```python
from build123d import *

# Parameters (mm, degrees)
SKETCH2_R          = 1.75
SKETCH2_R_2        = 4
SKETCH2_R_3        = 1
CUT_EXTRUDE5_DEPTH = 31.724582991
SKETCH2_7_R        = 10
CUT_EXTRUDE6_DEPTH = 7.5


with BuildPart() as part:
    # Sketch1 → Revolve2 (revolve)
    with BuildSketch(Plane.XY):
        Polygon((0, 12), (0, 0), (-20, 0), (-20, 5), (-17.5, 5), (-17.5, 12), align=None)
    revolve(axis=Axis((0, 12, 0), (0, -1, 0)))

    # Sketch2 → Cut-Extrude5 (cut, through all)
    with BuildSketch(Plane.XZ):
        with Locations((-7.340557342, -12.660927377)):
            Circle(SKETCH2_R)
        with Locations((14.5, 0)):
            Circle(SKETCH2_R)
        with Locations((-7.384963415, 12.584013803)):
            Circle(SKETCH2_R)
        Circle(SKETCH2_R_2)
        with Locations((0, 7)):
            Circle(SKETCH2_R_3)
        with Locations((-7, 0)):
            Circle(SKETCH2_R_3)
        with Locations((7, 0)):
            Circle(SKETCH2_R_3)
        with Locations((0, -7)):
            Circle(SKETCH2_R_3)
    extrude(amount=-CUT_EXTRUDE5_DEPTH, mode=Mode.SUBTRACT)

    # Sketch2_7 → Cut-Extrude6 (cut)
    with BuildSketch(Plane.XZ):
        Circle(SKETCH2_7_R)
    extrude(amount=-CUT_EXTRUDE6_DEPTH, mode=Mode.SUBTRACT)


solid = part.part
```
Here's how the part is built. I have some questions about the finished solid (model axes, mm). A direction names the side the tool comes from. Coordinates: 2 decimals unless noted, no trailing zeros. Loops run counter-clockwise (first coordinate to the right, second up) from the corner with the lowest first, then second, coordinate; pieces in that order, holes last. Notation, with made-up numbers: (-8.75, 18) - (-2.75, 18) arc R17 cw to (-2.75, 46) - close; hole circle Ø1 at (2.25, 32.25). An arc over 180 degrees is marked (long way). Return JSON: item names as keys, results as strings. Group by question number.
Item 1: On a 3-axis mill with a long thin cutter (end or side, diameter ignored), from which of +Z, -Z, +X, -X, +Y, -Y can I reach the whole of each face in a straight line? I mean faces 4 (the face through (13.887, 8.549, 10.648)), 5 (the face through (-0.1, 7.5, -4.3)), 6 (the face through (16.169, 5.916, 0.526)). Say none if no direction works.
Item 2: If we section it at C-C on y = 9.75: State how many separate pieces and enclosed holes the cut face has, and give its area (3 significant figures).
Item 3: If we section it at D-D on x = 7: Write out the boundary of the cut face in (y, z) (3 decimals), and give its area (3 significant figures).
Item 4: I need wall thicknesses on line 1 (Z direction, x = 0, y = 10.15); line 2 (Y direction, x = 3.5, z = 4); line 3 (X direction, y = 11.5, z = 1.5). Which ranges of each line are inside material? Lowest first, please. Write a range as from..to.
Item 5: Will these pins go through, and if not, where does the flat tip stop? P1, Ø16, axis at x = 0, z = 0, coming from the +Y side; P2, Ø2, axis at y = 8.5, z = 8, coming from the -X side; P3, Ø3, axis at y = 1.5, z = 9, coming from the -X side; P4, Ø10, axis at x = -0.5, z = -4.5, coming from the -Y side.
Item 6: If we section it at B-B on z = -12: Write out the boundary of the cut face in (x, y), and give its area (3 significant figures).
Item 7: If we section it at A-A on x = 0: Write out the boundary of the cut face in (y, z), and give its area (3 significant figures).
Item 8: We'd pull the mould along Z, two halves only. Please class faces 1 (the face through (4.336, 2.535, 19.524)), 2 (the face through (0, 10, 8)), 3 (the face through (-9, 0, -5)): +Z half, -Z half, draft (parallel to the pull), parting line (faces both ways), or undercut.
Calculated:
{
 "1": {"face 4": "+Y", "face 5": "-Y", "face 6": "+Y, -Y"},
 "2": {"separate pieces": "1", "enclosed holes": "8", "area": "870 mm^2"},
 "3": {"outline": "(0, -18.735) - (5, -18.735) - (5, -16.039) - (12, -16.039) - (12, -1) - (7.5, -1) - (7.5, -7.141) - (0, -7.141) - close; (0, 7.141) - (7.5, 7.141) - (7.5, 1) - (12, 1) - (12, 16.039) - (5, 16.039) - (5, 18.735) - (0, 18.735) - close", "area": "296 mm^2"},
 "4": {"line 1": "z = -17.5..-8, -6..-4, 4..6, 8..17.5", "line 2": "y = 7.5..12", "line 3": "x = -17.44..-3.71, 3.71..13.6, 15.4..17.44"},
 "5": {"P1": "stops at y = 12", "P2": "stops at x = -16.04", "P3": "stops at x = -18.54", "P4": "stops at y = 7.5"},
 "6": {"outline": "(-16, 0) - (-8.96, 0) - (-8.96, 12) - (-12.74, 12) - (-12.74, 5) - (-16, 5) - close; (-5.72, 0) - (16, 0) - (16, 5) - (12.74, 5) - (12.74, 12) - (-5.72, 12) - close", "area": "299 mm^2"},
 "7": {"outline": "(0, -20) - (5, -20) - (5, -17.5) - (12, -17.5) - (12, -8) - (7.5, -8) - (7.5, -10) - (0, -10) - close; (0, 10) - (7.5, 10) - (7.5, 8) - (12, 8) - (12, 17.5) - (5, 17.5) - (5, 20) - (0, 20) - close; (7.5, -6) - (12, -6) - (12, -4) - (7.5, -4) - close; (7.5, 4) - (12, 4) - (12, 6) - (7.5, 6) - close", "area": "241 mm^2"},
 "8": {"face 1": "parting line", "face 2": "undercut", "face 3": "draft"}
}
